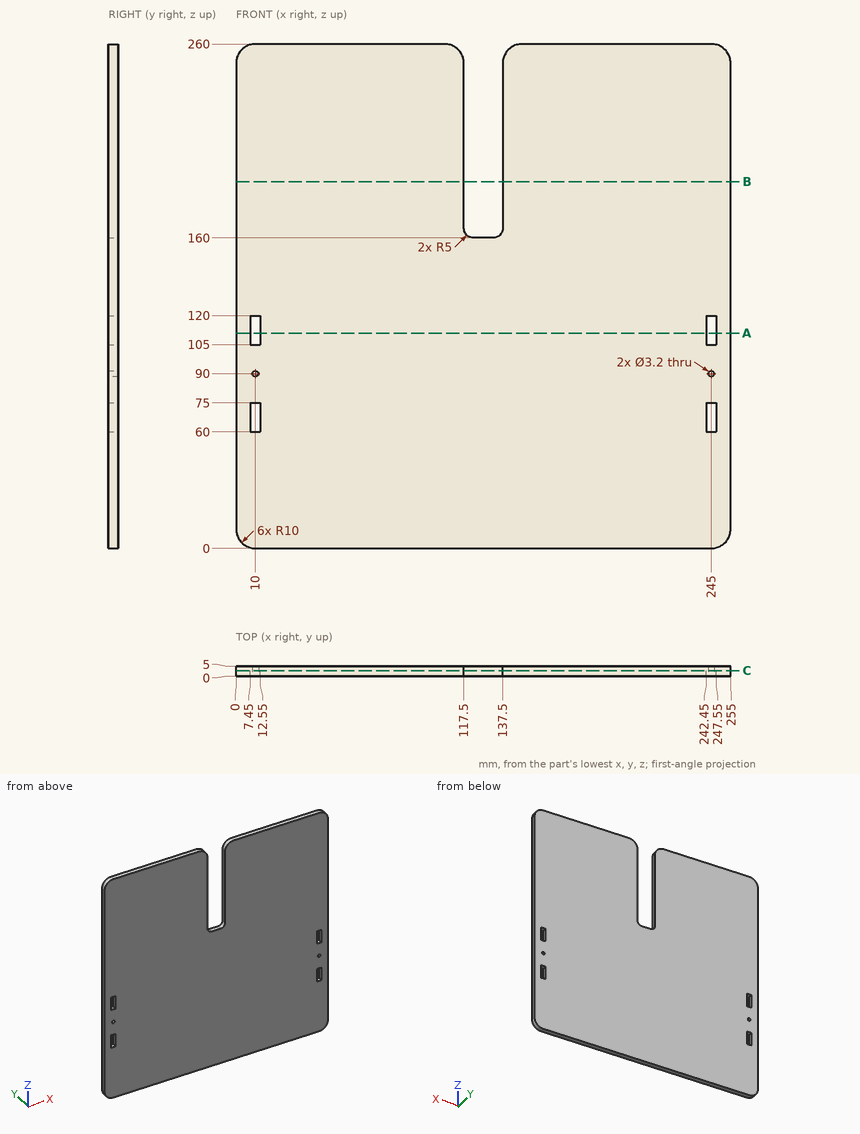
Verification items for this drawing (mm, ordinates from the low corner). Give positions to 0.01 mm unless a question says otherwise; leave off trailing zeros. Write each loop counter-clockwise with the first axis right and the second up, starting at its lowest first coordinate (ties: lowest second). Pieces come first, ordered by that corner, then holes. Notation, with made-up numbers: (71, 36) - (97, 36) arc R15 cw to (97, 50) - close; hole circle Ø6 at (30.25, 89.5). An arc over 180 degrees is marked (long way). Answer as a JSON object with one key per item and string values. Group by question number.
1) Depth check by flat-ended pin: P1, Ø3, axis at x = 245, z = 90, coming from the -Y side (3 decimals); P2, Ø1.5, axis at x = 132.5, y = 1.5, coming from the +Z side. Enter the tip coordinate at first touch or a pass-through.
2) Thickness scan on probe 1 along Z at (x, y) = (245, 1.8); probe 2 along X at (y, z) = (3.3, 73); probe 3 along X at (y, z) = (2.35, 90). Record the ranges inside material, lowest first. Write a range as from..to.
3) Sectioned sample at A-A (z = 111). Record the cut outline in (x, y).
4) Sectioned sample at C-C (y = 2.75). Give the number of separate pieces and of enclosed holes in the cut face, then the cut area to 3 significant figures.
5) Sectioned sample at B-B (z = 189). Record the cut outline in (x, y), then the cut area to 4 significant figures.
Geometry results:
{
 "1": {"P1": "passes through", "P2": "stops at z = 160.06"},
 "2": {"probe 1": "z = 0..60, 75..88.4, 91.6..105, 120..260", "probe 2": "x = 0..7.45, 12.55..242.45, 247.55..255", "probe 3": "x = 0..8.4, 11.6..243.4, 246.6..255"},
 "3": {"outline": "(0, 0) - (7.45, 0) - (7.45, 5) - (0, 5) - close; (12.55, 0) - (242.45, 0) - (242.45, 5) - (12.55, 5) - close; (247.55, 0) - (255, 0) - (255, 5) - (247.55, 5) - close"},
 "4": {"separate pieces": "1", "enclosed holes": "6", "area": "63,900 mm^2"},
 "5": {"outline": "(0, 0) - (117.5, 0) - (117.5, 5) - (0, 5) - close; (137.5, 0) - (255, 0) - (255, 5) - (137.5, 5) - close", "area": "1,175 mm^2"}
}
